Verification items for this drawing (mm, ordinates from the low corner). Round coordinates to 2 decimals unless told otherwise and drop trailing zeros. Write each loop counter-clockwise with the first axis right and the second up, starting at its lowest first coordinate (ties: lowest second). Pieces come first, ordered by that corner, then holes.
Item 1: Cross-section at A-A (y = 5.08). Enter the section's corners in (x, z), then the cut area to 3 significant figures.
Item 2: Cross-section at D-D (z = 15). Enter the section's corners in (x, y).
Item 3: Scan lines: probe 1 along Z at (x, y) = (5, 85) (1 decimal); probe 2 along Y at (x, z) = (0.5, 5); probe 3 along Y at (x, z) = (4.25, 30.5) (1 decimal). Record each from-to range of solid material in increasing order.
Item 4: Cross-section at C-C (y = 80). Enter the section's corners in (x, z).
Item 5: Cross-section at B-B (x = 2.25). State how many separate pieces and enclosed holes the cut face has, then the cut area to 3 significant figures.
Item 6: Draft check along Z on the marked faces 1, 2 and 3. Enter one of: pulls with the +Z half, pulls with the -Z half, needs draft (parallel to the pull), parting line crosses it, or undercut.
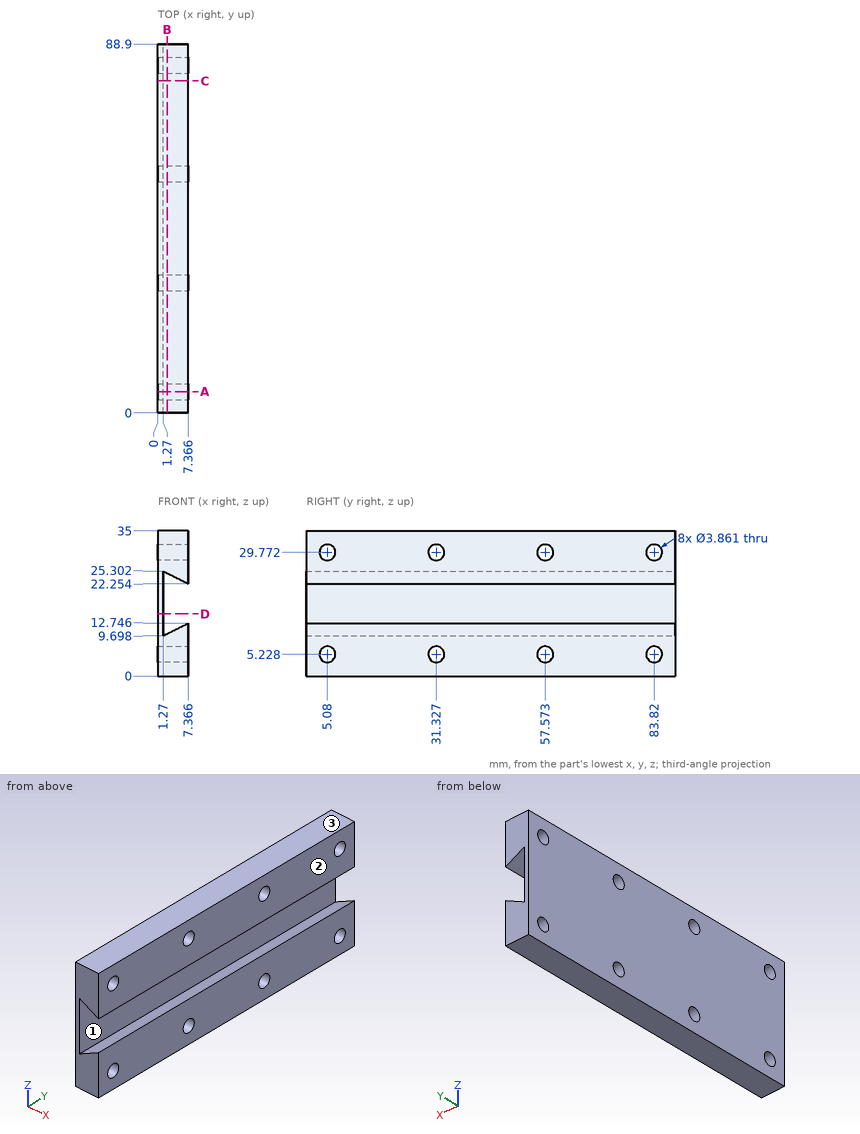
Resolved:
1. outline: (0, 0) - (7.37, 0) - (7.37, 3.3) - (0, 3.3) - close; (0, 7.16) - (7.37, 7.16) - (7.37, 12.75) - (1.27, 9.7) - (1.27, 25.3) - (7.37, 22.25) - (7.37, 27.84) - (0, 27.84) - close; (0, 31.7) - (7.37, 31.7) - (7.37, 35) - (0, 35) - close
1. area: 124 mm2
2. outline: (0, 0) - (1.27, 0) - (1.27, 88.9) - (0, 88.9) - close
3. probe 1: z = 0 to 3.7, 6.8 to 11.6, 23.4 to 28.2, 31.3 to 35
3. probe 2: y = 0 to 3.16, 7 to 29.41, 33.24 to 55.66, 59.49 to 81.9, 85.74 to 88.9
3. probe 3: y = 0 to 3.3, 6.9 to 29.5, 33.1 to 55.8, 59.4 to 82, 85.6 to 88.9
4. outline: (0, 0) - (7.37, 0) - (7.37, 12.75) - (1.27, 9.7) - (1.27, 25.3) - (7.37, 22.25) - (7.37, 35) - (0, 35) - close
5. separate pieces: 2
5. enclosed holes: 8
5. area: 1,720 mm2
6. face 1: undercut
6. face 2: needs draft
6. face 3: pulls with the +Z half
